Input: dimensioned drawing with shaded views. Units: mm. Origin: part minimum x, y, z. A direction names the side the tool comes from. Give positions to 0.01 mm unless a question says otherwise; leave off trailing zeros. Loops run counter-clockwise (first coordinate to the right, second up) from the corner with the lowest first, then second, coordinate; pieces in that order, holes last. Notation, with made-up numbers: M 14,-33 L 46,-33 A31 ccw 46,-7 Z; hole C 63.25,71 d11. An arc over 180 degrees is marked long. Answer in a Markdown table with one row per item.
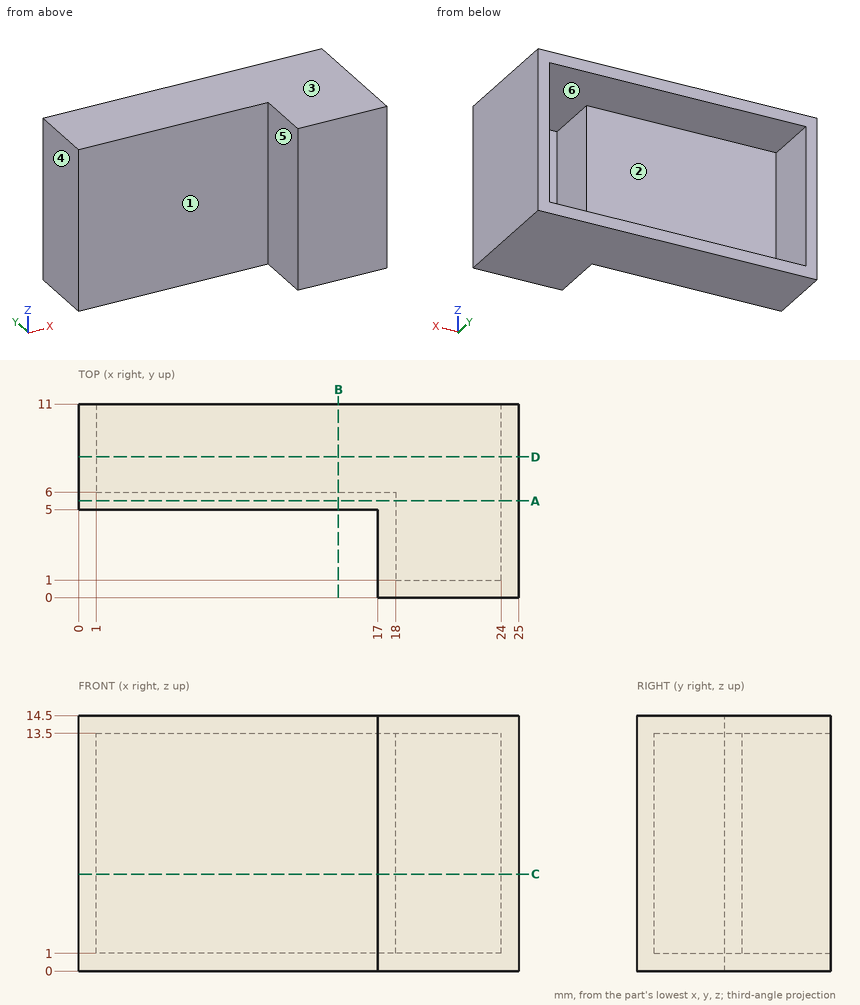
Q1. Contact query for flat-ended pins moving along their axis: pin 1 Ø5 at (y, z) = (7.5, 5.5) entering from -X; pin 2 Ø3 at (x, z) = (21.5, 9) entering from +Y; pin 3 Ø2.5 at (y, z) = (3, 5.5) entering from -X; pin 4 Ø6 at (x, z) = (11, 10) entering from +Y. Output: stop coordinate, or through.
Values follow:
| item | result |
|---|---|
| pin 1 | x = 0 |
| pin 2 | y = 1 |
| pin 3 | x = 17 |
| pin 4 | y = 6 |
Q2. Reachability of the marked faces 4, 5 and 6 from +Z, -Z, +X, -X, +Y, -Y: full face, straight path, thin tool, end or side. Return the list, or none.
Values follow:
| item | result |
|---|---|
| face 4 | +Z, -Z, -X, +Y, -Y |
| face 5 | +Z, -Z, -X, -Y |
| face 6 | +Y |
Q3. Section query D-D (y = 8). Output: boundary loops of the cut face in (x, z), plus the area to 3 significant figures.
Values follow:
| item | result |
|---|---|
| outline | M 0,0 L 25,0 L 25,14.5 L 0,14.5 Z; hole M 1,1 L 24,1 L 24,13.5 L 1,13.5 Z |
| area | 75.0 mm^2 |
Q4. Section query B-B (x = 14.75). Output: boundary loops of the cut face in (y, z), plus the area to 3 significant figures.
Values follow:
| item | result |
|---|---|
| outline | M 5,0 L 11,0 L 11,1 L 6,1 L 6,13.5 L 11,13.5 L 11,14.5 L 5,14.5 Z |
| area | 24.5 mm^2 |
Q5. Ray query, probe 1 along Z at (x, y) = (15.75, 8.5); probe 2 along X at (y, z) = (1.5, 6.25); probe 3 along X at (y, z) = (8.5, 3). Return the intervals inside material, ascending. Write a range as from..to.
Values follow:
| item | result |
|---|---|
| probe 1 | 0..1, 13.5..14.5 |
| probe 2 | 17..18, 24..25 |
| probe 3 | 0..1, 24..25 |
Q6. Section query A-A (y = 5.5). Output: boundary loops of the cut face in (x, z), plus the area to 4 significant figures.
Values follow:
| item | result |
|---|---|
| outline | M 0,0 L 25,0 L 25,14.5 L 0,14.5 Z; hole M 18,1 L 24,1 L 24,13.5 L 18,13.5 Z |
| area | 287.5 mm^2 |
Q7. Mould query, pull axis Z, two halves, no side actions, for the marked faces 1, 2 and 3. Classes: +Z half, -Z half, draft (parallel to the pull), parting line (faces both ways), or undercut.
Values follow:
| item | result |
|---|---|
| face 1 | draft |
| face 2 | undercut |
| face 3 | +Z half |
Q8. Section query C-C (z = 5.5). Output: boundary loops of the cut face in (x, y).
Values follow:
| item | result |
|---|---|
| outline | M 0,5 L 17,5 L 17,0 L 25,0 L 25,11 L 24,11 L 24,1 L 18,1 L 18,6 L 1,6 L 1,11 L 0,11 Z |
